Drawing for the job (mm, zero at the part's lowest x, y, z). A direction names the side the tool comes from. Round coordinates to 2 decimals unless told otherwise and drop trailing zeros. Loops run counter-clockwise (first coordinate to the right, second up) from the corner with the lowest first, then second, coordinate; pieces in that order, holes last. Notation, with made-up numbers: (61, 71.5) - (90, 71.5) arc R19 cw to (90, 107.5) - close; hole circle Ø2 at (-13.5, -39.75). An arc over 180 degrees is marked (long way). Put each result on its own line as item: value.
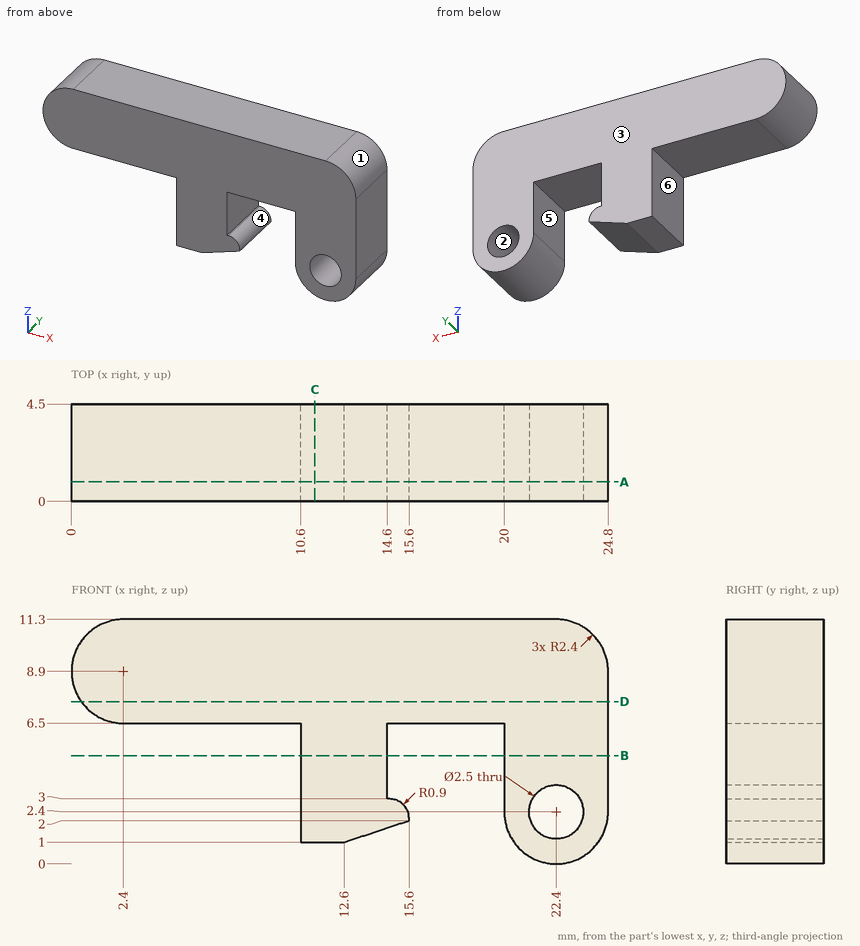
1. Two-plate mould, pull along Z, no slides. Class the marked faces 1, 2 and 3: pulls with the +Z half, pulls with the -Z half, needs draft (parallel to the pull), parting line crosses it, or undercut.
A:
face 1: pulls with the +Z half
face 2: undercut
face 3: needs draft
2. Band-saw the part on D-D (z = 7.5). List the corners of the cut face in (x, y).
A:
outline: (0.45, 0) - (24.8, 0) - (24.8, 4.5) - (0.45, 4.5) - close
3. Probe line 1 along X through (y, z) = (1.95, 2.4); line 2 along X through (y, z) = (0.85, 4.25); line 3 along Z through (x, y) = (15.25, 3.2). List the from-to ranges inside material, lowest first. Write a range as [from, to].
A:
line 1: x = [10.6, 15.55], [20, 21.15], [23.65, 24.8]
line 2: x = [10.6, 14.6], [20, 24.8]
line 3: z = [1.88, 2.81], [6.5, 11.3]
4. Pin check, flat tips, straight feed: P1, Ø1.3, axis at x = 6.5, y = 2.5, coming from the -Z side; P2, Ø1.5, axis at x = 17.5, z = 5.5, coming from the -Y side; P3, Ø1.3, axis at y = 3, z = 4.5, coming from the -X side; P4, Ø2, axis at x = 11.5, y = 4, coming from the -Z side. Stop position of each tip, or through.
A:
P1: stops at z = 6.5
P2: passes through
P3: stops at x = 10.6
P4: stops at z = 1
5. Band-saw the part on C-C (x = 11.25). List the corners of the cut face in (y, z), plus the area to 4 significant figures.
A:
outline: (0, 1) - (4.5, 1) - (4.5, 11.3) - (0, 11.3) - close
area: 46.35 mm²
6. Band-saw the part on A-A (y = 0.9). List the corners of the cut face in (x, z).
A:
outline: (2.4, 6.5) - (10.6, 6.5) - (10.6, 1) - (12.6, 1) - (15.6, 2) - (15.6, 2.1) arc R0.9 ccw to (14.7, 3) - (14.6, 3) - (14.6, 6.5) - (20, 6.5) - (20, 2.4) arc R2.4 ccw to (24.8, 2.4) - (24.8, 8.9) arc R2.4 ccw to (22.4, 11.3) - (2.4, 11.3) arc R2.4 ccw to start; hole circle Ø2.5 at (22.4, 2.4)
7. Band-saw the part on B-B (z = 5). List the corners of the cut face in (x, y).
A:
outline: (10.6, 0) - (14.6, 0) - (14.6, 4.5) - (10.6, 4.5) - close; (20, 0) - (24.8, 0) - (24.8, 4.5) - (20, 4.5) - close
8. Tool access for the marked faces 4, 5 and 6: list every direction of +Z, -Z, +X, -X, +Y, -Y with a clear straight run to the whole face (end or side of a thin tool).
A:
face 4: +Y, -Y
face 5: -Z, +Y, -Y
face 6: -Z, -X, +Y, -Y
